Autodesk Inventor part; units mm, degrees
ref_plane "YZ Plane" through (0, 0, 0) normal (1, 0, 0) x (0, 1, 0)
ref_plane "XZ Plane" through (0, 0, 0) normal (0, 1, 0) x (-1, 0, 0)
ref_plane "XY Plane" through (0, 0, 0) normal (0, 0, 1) x (1, 0, 0)
sketch "Sketch1" plane through (0, 0, 0) normal (0, 0, 1) x (1, 0, 0)
  line L0 (0, 0) -> (7.3125, 0)
  line L1 (7.3125, 0) -> (7.3125, 17.7174)
  line L2 (7.3125, 17.7174) -> (0, 17.7174)
  line L3 (0, 17.7174) -> (0, 0)
extrude "Extrusion1" add sketch "Sketch1" along normal blind 6.5
sketch "Sketch2" plane through (0, 17.7174, 0) normal (0, 1, 0) x (1, 0, 0)
  line L0 (7.3125, 0) -> (0, 0)
  line L1 (0, 0) -> (0, -6.5)
  line L2 (7.3125, -6.5) -> (0, -6.5)
  line L3 (7.3125, 0) -> (7.3125, -6.5)
  circle A0 centre (3.6562, -3.25) radius 1.8618
extrude "Extrusion2" add sketch "Sketch2" along normal blind 11.5 contours A0
ref_plane "Work Plane1" through (0, 0, 3.25) normal (0, 0, 1) x (1, 0, 0)
sketch "Sketch3" plane through (0, 0, 3.25) normal (0, 0, 1) x (1, 0, 0)
  line L0 (5.5181, 29.2174) -> (1.7944, 29.2174)
  spline S0 degree 4 poles (3.6562, 29.2174) (1.2604, 37.8636) (7.2009, 60.1511) (32.7256, 44.0854) (31.2731, 30.1217) knots 0 0 0 0 0 1 1 1 1 1
  point P0 (0, 0)
  point P1 (4.4619, 39.176)
  point P2 (11.5543, 46.3185)
  point P3 (23.5265, 44.0553)
sketch "Sketch4" plane through (3.6562, 29.2174, 3.25) normal (0, 1, 0) x (1, 0, 0)
  circle A0 centre (0, 0) radius 1.8618
  point P0 (-3.6562, 3.25)
sweep "Sweep1" add profiles "Sketch4" path "Sketch3" path curves S0
sketch "Sketch5" plane through (0, 0, 6.5) normal (0, 0, 1) x (1, 0, 0)
  line L0 (0, 17.7174) -> (0, 0)
  line L1 (7.3125, 0) -> (7.3125, 17.7174)
  line L2 (0, 0) -> (7.3125, 0)
  line L3 (7.3125, 0) -> (7.3125, 7.8965)
  line L4 (7.3125, 7.8965) -> (0, 7.8965)
  line L5 (0, 7.8965) -> (0, 0)
extrude "Extrusion3" add sketch "Sketch5" along normal blind 8.25
sketch "Sketch6" plane through (0, 0, 14.75) normal (0, 0, 1) x (1, 0, 0)
  circle A0 centre (3.6562, 3.9482) radius 2.358
  line L0 (7.3125, 7.8965) -> (0, 7.8965)
  line L1 (0, 7.8965) -> (0, 0)
  line L2 (0, 0) -> (7.3125, 0)
  line L3 (7.3125, 0) -> (7.3125, 7.8965)
  point P0 (7.3125, 3.9482)
  point P1 (3.6562, 0)
extrude "Extrusion4" cut sketch "Sketch6" against normal through all contours A0
sketch "Sketch7" plane through (7.3125, 0, 0) normal (1, 0, 0) x (0, 0, -1)
  line L0 (0, 0) -> (0, 17.7174)
  line L1 (0, 17.7174) -> (-6.5, 17.7174)
  line L2 (-6.5, 7.8965) -> (-6.5, 17.7174)
  line L3 (-6.5, 7.8965) -> (-14.75, 7.8965)
  line L4 (-14.75, 0) -> (-14.75, 7.8965)
  line L5 (0, 0) -> (-14.75, 0)
  circle A0 centre (-10.625, 4.3798) radius 1.7093
extrude "Extrusion5" cut sketch "Sketch7" against normal up to next contours A0
properties part number "platformHookv1"
Input: part model. Units: mm. Frame: model coordinates. A direction names the side the tool comes from. Round coordinates to 2 decimals unless told otherwise and drop trailing zeros. Loops run counter-clockwise (first coordinate to the right, second up) from the corner with the lowest first, then second, coordinate; pieces in that order, holes last. Notation, with made-up numbers: (-33.5, 57) -> (20.5, 57) arc R31 cw to (20.5, 83) -> close; hole circle Ø5 at (41.25, -17). An arc over 180 degrees is marked (long way). Answer as a JSON object with one key per item and string values. Group by question number.
1) Section query B-B on y = 21. Output: boundary loops of the cut face in (x, z).
2) Draft query along Y for faces 4 (the flat face through (4, 9, 0)), 5 (the flat face through (4, 7.896, 11)), 6 (the flat face through (4, 0, 7)), 7 (the cylindrical face through (1.3, 4.05, 7.48)). Return one class per face: +Y half, -Y half, draft (parallel to the pull), parting line (faces both ways), or undercut.
3) Section query A-A on z = 7.5. Output: boundary loops of the cut face in (x, y), plus the area to 3 significant figures.
4) Ray query, L1, parallel to X at y = 8.5, z = 1.25; L2, parallel to X at y = 3, z = 12; L3, parallel to Z at x = 4, y = 37. Return the intervals inside material, ascending.
5) Section query C-C on z = 11.75. Output: boundary loops of the cut face in (x, y).
6) Pin query (flat end, axial travel): pin 1 (8 mm diameter, centred on x = 5, z = 10, fed in from +Y); pin 2 (6 mm diameter, centred on x = 3.66, y = 3.95, fed in from -Z); pin 3 (3 mm diameter, centred on x = 4.5, y = 21.5, fed in from -Z); pin 4 (5.5 mm diameter, centred on y = 4.38, z = 10.62, fed in from +X). Return the tip coordinate at first contact, or that it passes through.
7) Reachability of faces 1 (the flat face through (4, 13, 6.5)), 2 (the flat face through (7.312, 7, 6)), 3 (the flat face through (31.12, 30.18, 3.23)) from +Z, -Z, +X, -X, +Y, -Y: full face, straight path, thin tool, end or side. Return the list, or none.
Reply:
{
 "1": {"outline": "circle Ø3.72 at (3.66, 3.25)"},
 "2": {"face 4": "draft", "face 5": "+Y half", "face 6": "-Y half", "face 7": "undercut"},
 "3": {"outline": "(0, 0) -> (7.31, 0) -> (7.31, 7.9) -> (0, 7.9) -> close; hole circle Ø4.72 at (3.66, 3.95)", "area": "40.3 mm2"},
 "4": {"L1": "x = 0 to 7.31", "L2": "x = 0 to 1.5, 5.82 to 7.31", "L3": "z = 1.4 to 5.1"},
 "5": {"outline": "(0, 0) -> (7.31, 0) -> (7.31, 3.09) -> (5.85, 3.09) arc R2.36 cw (long way) to (5.27, 5.67) -> (7.31, 5.67) -> (7.31, 7.9) -> (0, 7.9) -> close"},
 "6": {"pin 1": "stops at y = 17.72", "pin 2": "stops at z = 0", "pin 3": "stops at z = 1.39", "pin 4": "stops at x = 7.31"},
 "7": {"face 1": "+Z, +X, -X, +Y", "face 2": "+Z, -Z, +X, -Y", "face 3": "+Z, -Z, -Y"}
}
